Design review of the part built by this model. Coordinates are the model's own, in mm. A direction names the side the tool comes from. Give positions to 0.01 mm unless a question says otherwise; leave off trailing zeros. Write each loop counter-clockwise with the first axis right and the second up, starting at its lowest first coordinate (ties: lowest second). Pieces come first, ordered by that corner, then holes. Notation, with made-up numbers: M 59,85 L 92,85 A14 cw 92,104 Z; hole C 36.25,36 d5. An arc over 180 degrees is marked long. Write each question's results on one line, items separated by ' | '. Start each with the question number.
from build123d import *

# Parameters (mm, degrees)
SKETCH_1_W          = 46.5
SKETCH_1_H          = 57.5
EXTRUDE_1_DEPTH     = 1.6
SKETCH_2_W          = 46.5
SKETCH_2_H          = 57.5
SKETCH_2_W_2        = 13.15
SKETCH_2_H_2        = 54.1
SKETCH_2_W_3        = 15
EXTRUDE_2_DEPTH     = 15.3
SKETCH_3_R          = 1.5
CUT_EXTRUDE_1_DEPTH = 41.653843607
CUT_EXTRUDE_START   = -1.6
SKETCH_3_3_R        = 2.5
CUT_EXTRUDE_2_DEPTH = 0.8


with BuildPart() as part:
    # 草图1 → 凸台-拉伸1 (new body)
    with BuildSketch(Plane(origin=(0, 0, 0), x_dir=(1, 0, 0), z_dir=(0, 1, 0))):
        Rectangle(SKETCH_1_W, SKETCH_1_H)
    extrude(amount=EXTRUDE_1_DEPTH)

    # 草图2 → 凸台-拉伸2 (add)
    with BuildSketch(Plane(origin=(0, 1.6, 0), x_dir=(1, 0, 0), z_dir=(0, 1, 0))):
        Rectangle(SKETCH_2_W, SKETCH_2_H)
        with Locations((-15.375, 0)):
            Rectangle(SKETCH_2_W_2, SKETCH_2_H_2, mode=Mode.SUBTRACT)
        Rectangle(SKETCH_2_W_3, SKETCH_2_H_2, mode=Mode.SUBTRACT)
        with Locations((15.375, 0)):
            Rectangle(SKETCH_2_W_2, SKETCH_2_H_2, mode=Mode.SUBTRACT)
    extrude(amount=EXTRUDE_2_DEPTH)

    # 草图3 → 切除-拉伸1 (cut, through all)
    with BuildSketch(Plane.XZ):
        with Locations(Location((-15.1, 0, 0), (0, 0, 270))):
            Circle(SKETCH_3_R)
        with Locations(Location((15.1, 0, 0), (0, 0, 270))):
            Circle(SKETCH_3_R)
    extrude(amount=-CUT_EXTRUDE_1_DEPTH, mode=Mode.SUBTRACT)

    # 草图3<3> → 切除-拉伸2 (cut)
    with BuildSketch(Plane.XZ.offset(CUT_EXTRUDE_START)):
        with Locations(Location((-15.1, 0, 0), (0, 0, 90))):
            Circle(SKETCH_3_3_R)
        with Locations(Location((15.1, 0, 0), (0, 0, 90))):
            Circle(SKETCH_3_3_R)
    extrude(amount=CUT_EXTRUDE_2_DEPTH, mode=Mode.SUBTRACT)


solid = part.part
Q1. For faces 1 (the flat face through (15, 9, 27.05)), 2 (the cylindrical face through (16.587, 0.394, 0.195)), list the 3-axis set-ups (+Z, -Z, +X, -X, +Y, -Y) from which the entire face can be reached by the end or side of a thin tool; tool diameter is ignored.
Q2. Wall thickness on line 1 along X through (y, z) = (1.2, 0); line 2 along X through (y, z) = (11.25, 4); line 3 along Z through (x, y) = (-20.5, 5.25): over which ranges is each line inside the solid? List them lowest first. Write a range as from..to.
Q3. We need section B-B on z = 0. Count the separate pieces of the cut face and the enclosed holes in it, and give its area (3 significant figures).
Q4. For pin 1 Ø5.5 at (x, z) = (14.5, -0.5) entering from +Y; pin 2 Ø2.5 at (x, z) = (-15.1, 0) entering from -Y, all flat-tipped, find the tip position at first contact; note any pin that passes through.
Q5. The part is to be moulded in two halves that separate along Z. For faces 3 (the flat face through (0, 9, 27.05)), 4 (the flat face through (8.5, 16.9, -0.1)), 5 (the flat face through (0, 8, 28.75)), 6 (the flat face through (-7.5, 9, 0)), say which applies: pulls with the +Z half, pulls with the -Z half, needs draft (parallel to the pull), parting line crosses it, or undercut.
Q6. We need section C-C on y = 4.5. Write out the cut boundary in (x, z).
Q7. We need section D-D on x = 0. Write out the cut boundary in (y, z), and give its area (3 significant figures).
Q8. We need section A-A on x = -15.1. Write out the cut boundary in (y, z), and give its area (3 significant figures).
Answer sheet:
1) face 1: +Y | face 2: +Y, -Y
2) line 1: -23.25..-17.6, -12.6..12.6, 17.6..23.25 | line 2: -23.25..-21.95, -8.8..-7.5, 7.5..8.8, 21.95..23.25 | line 3: -28.75..-27.05, 27.05..28.75
3) separate pieces: 3 | enclosed holes: 0 | area: 141 mm^2
4) pin 1: y = 1.6 | pin 2: through
5) face 3: undercut | face 4: needs draft | face 5: pulls with the +Z half | face 6: undercut
6) outline: M -23.25,-28.75 L 23.25,-28.75 L 23.25,28.75 L -23.25,28.75 Z; hole M -21.95,-27.05 L -8.8,-27.05 L -8.8,27.05 L -21.95,27.05 Z; hole M -7.5,-27.05 L 7.5,-27.05 L 7.5,27.05 L -7.5,27.05 Z; hole M 8.8,-27.05 L 21.95,-27.05 L 21.95,27.05 L 8.8,27.05 Z
7) outline: M 0,-28.75 L 16.9,-28.75 L 16.9,-27.05 L 1.6,-27.05 L 1.6,27.05 L 16.9,27.05 L 16.9,28.75 L 0,28.75 Z | area: 144 mm^2
8) outline: M 0,-28.75 L 16.9,-28.75 L 16.9,-27.05 L 1.6,-27.05 L 1.6,-2.5 L 0.8,-2.5 L 0.8,-1.5 L 0,-1.5 Z; M 0,1.5 L 0.8,1.5 L 0.8,2.5 L 1.6,2.5 L 1.6,27.05 L 16.9,27.05 L 16.9,28.75 L 0,28.75 Z | area: 138 mm^2
